CAD build for the part. Positions are in the model's coordinates, mm. A direction names the side the tool comes from. Round coordinates to 2 decimals unless told otherwise and drop trailing zeros. Loops run counter-clockwise (first coordinate to the right, second up) from the corner with the lowest first, then second, coordinate; pieces in that order, holes last.
from build123d import *

# Parameters (mm, degrees)
F0_R     = 3.048
F1_DEPTH = 152.4
F2_R     = 2.38125
F3_DEPTH = 0.79375
F4_R     = 1.5875
F5_DEPTH = 3.175
F7_DEPTH = 25.4


with BuildPart() as f1:
    # F0 (on Top) → F1 (new body)
    with BuildSketch(Plane.XY):
        Circle(F0_R)
    extrude(amount=F1_DEPTH)

    # F2 (on face) → F3 (join)
    with BuildSketch(Plane.XY.offset(152.4)):
        Circle(F2_R)
    extrude(amount=F3_DEPTH)

    # F4 (on face) → F5 (join)
    with BuildSketch(Plane.XY.offset(153.19375)):
        Circle(F4_R)
    extrude(amount=F5_DEPTH)

    # F6 (on face) → F7 (join)
    with BuildSketch(Plane(origin=(0, 0, 0), x_dir=(1, 0, 0), z_dir=(0, 0, -1))):
        with BuildLine():
            Line((-1.245454, -1.755775), (1.245454, -1.755775))
            ThreePointArc((1.245454, -1.755775), (0, 2.15265), (-1.245454, -1.755775))
        make_face()
    extrude(amount=F7_DEPTH)


solid = f1.part
Item 1: 3-axis set-ups, long thin cutter, end or side, ignore diameter. For faces 1 (the flat face through (0, 0, -25.4)), 2 (the cylindrical face through (-0.34, -1.55, 154.76)), 3 (the cylindrical face through (0.08, -2.15, -12.52)): which of +Z, -Z, +X, -X, +Y, -Y reach the whole face in a straight line?
Verdict:
face 1: -Z, +X, -X, +Y, -Y
face 2: +Z
face 3: -Z
Item 2: Cut at B-B (y = 0). List the corners of the cut face in (x, z), plus the area to 3 significant figures.
Verdict:
outline: (-3.05, 0) - (-2.15, 0) - (-2.15, -25.4) - (2.15, -25.4) - (2.15, 0) - (3.05, 0) - (3.05, 152.4) - (2.38, 152.4) - (2.38, 153.19) - (1.59, 153.19) - (1.59, 156.37) - (-1.59, 156.37) - (-1.59, 153.19) - (-2.38, 153.19) - (-2.38, 152.4) - (-3.05, 152.4) - close
area: 1,050 mm2
Item 3: Cut at C-C (z = 91.5). List the corners of the cut face in (x, y).
Verdict:
outline: circle Ø6.1 at (0, 0)
Item 4: Wall check: L1, parallel to Z at x = -1.5, y = 1.5; L2, parallel to Z at x = 1.5, y = -2.25; L3, parallel to Y at x = -0.25, z = 45.5. Give the ranges that are in metal, low to high.
Verdict:
L1: z = -25.4 to 153.19
L2: z = 0 to 152.4
L3: y = -3.04 to 3.04
Item 5: Flat gauge pins, fed straight in: P1, Ø2, axis at x = -0.5, z = 134, coming from the -Y side; P2, Ø2, axis at x = -0.5, z = -16, coming from the +Y side; P3, Ø3, axis at y = -2.5, z = 21.5, coming from the -X side; P4, Ø1.5, axis at x = -1, z = 80, coming from the +Y side. Where does each tip first touch, or does it go through?
Verdict:
P1: stops at y = -3.05
P2: stops at y = 1.76
P3: stops at x = -2.88
P4: stops at y = 3.04
Item 6: Cut at A-A (x = 0). List the corners of the cut face in (y, z), plus the area to 3 significant figures.
Verdict:
outline: (-3.05, 0) - (-2.15, 0) - (-2.15, -25.4) - (1.76, -25.4) - (1.76, 0) - (3.05, 0) - (3.05, 152.4) - (2.38, 152.4) - (2.38, 153.19) - (1.59, 153.19) - (1.59, 156.37) - (-1.59, 156.37) - (-1.59, 153.19) - (-2.38, 153.19) - (-2.38, 152.4) - (-3.05, 152.4) - close
area: 1,040 mm2
